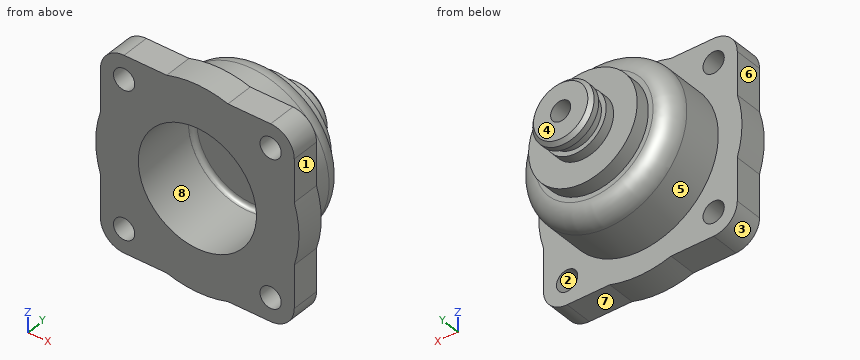
from build123d import *

# Parameters (mm, degrees)
SKETCH_1_R          = 4.5
EXTRUDE_1_DEPTH     = 12
FILLET_1_R          = 8
SKETCH_3_R          = 25
CUT_EXTRUDE_1_DEPTH = 29
FILLET_2_R          = 2
HOLE_WIZARD_M10_1_D = 8.5


with BuildPart() as part:
    # 草图1 → 凸台-拉伸1 (new body)
    with BuildSketch(Plane(origin=(0, 0, 0), x_dir=(1, 0, 0), z_dir=(0, 1, 0))):
        with BuildLine():
            Line((-41, 12.961481397), (-41, 31))
            ThreePointArc((-41, 31), (-38.071067812, 38.071067812), (-31, 41))
            Line((-31, 41), (-12.961481397, 41))
            ThreePointArc((-12.961481397, 41), (0, 43), (12.961481397, 41))
            Line((12.961481397, 41), (31, 41))
            ThreePointArc((31, 41), (38.071067812, 38.071067812), (41, 31))
            Line((41, 31), (41, 12.961481397))
            ThreePointArc((41, 12.961481397), (43, 0), (41, -12.961481397))
            Line((41, -12.961481397), (41, -31))
            ThreePointArc((41, -31), (38.071067812, -38.071067812), (31, -41))
            Line((31, -41), (12.961481397, -41))
            ThreePointArc((12.961481397, -41), (0, -43), (-12.961481397, -41))
            Line((-12.961481397, -41), (-31, -41))
            ThreePointArc((-31, -41), (-38.071067812, -38.071067812), (-41, -31))
            Line((-41, -31), (-41, -12.961481397))
            ThreePointArc((-41, -12.961481397), (-43, 0), (-41, 12.961481397))
        make_face()
        with Locations(Location((-31, 31, 0), (0, 0, 270))):
            Circle(SKETCH_1_R, mode=Mode.SUBTRACT)
        with Locations(Location((31, 31, 0), (0, 0, 270))):
            Circle(SKETCH_1_R, mode=Mode.SUBTRACT)
        with Locations(Location((31, -31, 0), (0, 0, 270))):
            Circle(SKETCH_1_R, mode=Mode.SUBTRACT)
        with Locations(Location((-31, -31, 0), (0, 0, 270))):
            Circle(SKETCH_1_R, mode=Mode.SUBTRACT)
    extrude(amount=EXTRUDE_1_DEPTH)

    # 草图2 → 旋转1 (revolve)
    with BuildSketch(Plane.XY):
        Polygon((0, 12), (33, 12), (33, 37), (23, 37), (23, 43), (13, 43), (13, 47), (11, 47), (11, 51), (13, 51), (13, 53.5), (11.5, 55), (0, 55), align=None)
    revolve(axis=Axis((0, 12, 0), (0, 1, 0)))

    # 圆角1
    fillet_1_edges = [part.edges().sort_by_distance(p)[0] for p in [
        (-33, 37, 0),
    ]]
    fillet(fillet_1_edges, radius=FILLET_1_R)

    # 草图3 → 切除-拉伸1 (cut)
    with BuildSketch(Plane.XZ):
        with Locations(Location((0, 0, 0), (0, 0, 270))):
            Circle(SKETCH_3_R)
    extrude(amount=-CUT_EXTRUDE_1_DEPTH, mode=Mode.SUBTRACT)

    # 圆角2
    fillet_2_edges = [part.edges().sort_by_distance(p)[0] for p in [
        (0, 29, 25),
    ]]
    fillet(fillet_2_edges, radius=FILLET_2_R)

    # M10 螺纹孔1 (through all)
    with Locations(Plane(origin=(0, 55, 0), x_dir=(1, 0, 0), z_dir=(0, 1, 0))):
        with Locations((0, 0)):
            Hole(HOLE_WIZARD_M10_1_D / 2)


solid = part.part
Geometry: final body of the model. Coordinates: model frame, mm. Face numbers are marked on the shaded views. A direction names the side the tool comes from. Round coordinates to 2 decimals unless told otherwise and drop trailing zeros. Order: outer loops, then holes, each group sorted by start corner. A loop starts at its lowest first (then second) coordinate and runs counter-clockwise, first axis right, second up. Notation, with made-up numbers: (30, -6.75) -> (43, -6.75) arc R25 cw to (43, 15.25) -> close; hole circle Ø1 at (79, 89). An arc over 180 degrees is marked (long way). Put each result on its own line as item: value. Start each with the question number.
Q1. Reachability of the marked faces 5, 6, 7 and 8 from +Z, -Z, +X, -X, +Y, -Y: full face, straight path, thin tool, end or side. Return the list, or none.
Q2. Section B-B on z = 28. Give the number of separate pieces and of enclosed holes in the cut face, and give its area (3 significant figures).
Q3. Line query: probe 1 along X at (y, z) = (8, -31); probe 2 along X at (y, z) = (9.5, -32); probe 3 along Y at (x, z) = (4, 7). Output: solid intervals per line, ascending.
Q4. First-contact query: pin 1 (8 mm diameter, centred on x = 0, z = -32.5, fed in from +Y); pin 2 (13 mm diameter, centred on x = -23.5, y = 5.5, fed in from -Z); pin 3 (3.5 mm diameter, centred on x = -22, y = 8.5, fed in from +Z). Flat tips, straight axial feed; report the tip coordinate or a pass-through.
Q5. Pull-direction query (X, two-part tool) for the marked faces 1, 2, 3 and 4; classes: +X half, -X half, draft (parallel to the pull), parting line (faces both ways), or undercut.
Q6. Section C-C on y = 30.5. Return the cut outline in (x, z).
Q7. Section A-A on y = 49.5. Return the cut outline in (x, z), and give its area (3 significant figures).
Ans:
1. face 5: +Y
1. face 6: +Z, -X, +Y, -Y
1. face 7: -Z, +X, +Y, -Y
1. face 8: -Y
2. separate pieces: 3
2. enclosed holes: 0
2. area: 1,630 mm2
3. probe 1: x = -41 to -35.5, -26.5 to 26.5, 35.5 to 41
3. probe 2: x = -40.95 to -35.39, -26.61 to 26.61, 35.39 to 40.95
3. probe 3: y = 29 to 55
4. pin 1: stops at y = 36.19
4. pin 2: stops at z = -41
4. pin 3: stops at z = 41
5. face 1: +X half
5. face 2: undercut
5. face 3: -X half
5. face 4: draft
6. outline: circle Ø65.72 at (0, 0); hole circle Ø8.5 at (0, 0)
7. outline: circle Ø22 at (0, 0); hole circle Ø8.5 at (0, 0)
7. area: 323 mm2
